Verification items for the finished model (mm, model axes). Round coordinates to 2 decimals unless told otherwise and drop trailing zeros. Order: outer loops, then holes, each group sorted by start corner. A loop starts at its lowest first (then second) coordinate and runs counter-clockwise, first axis right, second up. Notation, with made-up numbers: M 55.5,56 L 77.5,56 A19 cw 77.5,60 Z; hole C 37,-8.75 d11. An arc over 180 degrees is marked long. One line per item, written item: value. Start each with the question number.
from build123d import *

# Parameters (mm, degrees)
SKETCH009_W   = 75
SKETCH009_H   = 95
PAD005_DEPTH  = 3
SKETCH010_W   = 75
SKETCH010_H   = 95
SKETCH010_W_2 = 51.4
SKETCH010_H_2 = 20.2
SKETCH010_W_3 = 20
SKETCH010_H_3 = 92.6
SKETCH010_W_4 = 15.2
SKETCH010_H_4 = 35
SKETCH010_W_5 = 35
PAD006_DEPTH  = 30
FILLET003_R   = 1.8


with BuildPart() as part:
    # Sketch009 → Pad005 (new body)
    with BuildSketch(Plane.XZ):
        Rectangle(SKETCH009_W, SKETCH009_H)
    extrude(amount=PAD005_DEPTH)

    # Sketch010 → Pad006 (join)
    with BuildSketch(Plane.XZ.offset(2)):
        Rectangle(SKETCH010_W, SKETCH010_H)
        with Locations((-10.6, 36.2)):
            Rectangle(SKETCH010_W_2, SKETCH010_H_2, mode=Mode.SUBTRACT)
        with Locations((26.3, 0)):
            Rectangle(SKETCH010_W_3, SKETCH010_H_3, mode=Mode.SUBTRACT)
        with Locations((-28.7, 7.4)):
            Rectangle(SKETCH010_W_4, SKETCH010_H_4, mode=Mode.SUBTRACT)
        with Locations((-28.7, -28.8)):
            Rectangle(SKETCH010_W_4, SKETCH010_H_4, mode=Mode.SUBTRACT)
        with Locations((-2.4, 7.4)):
            Rectangle(SKETCH010_W_5, SKETCH010_H_4, mode=Mode.SUBTRACT)
        with Locations((-2.4, -28.8)):
            Rectangle(SKETCH010_W_5, SKETCH010_H_4, mode=Mode.SUBTRACT)
    extrude(amount=PAD006_DEPTH)

    # Fillet003
    fillet003_edges = [part.edges().sort_by_distance(p)[0] for p in [
        (0, 0, 47.5),
        (37.5, 0, 0),
        (0, 0, -47.5),
        (-37.5, 0, 0),
    ]]
    fillet(fillet003_edges, radius=FILLET003_R)


solid = part.part
1. Section check B-B (x = 30.5). Record the cut outline in (y, z), and give its area (3 significant figures).
2. Section check D-D (x = -3). Record the cut outline in (y, z), and give its area (3 significant figures).
3. Scan lines: line 1 along X through (y, z) = (-20, 8.5); line 2 along Z through (x, y) = (-29, -26); line 3 along X through (y, z) = (-12.5, 36). Record each from-to range of solid material in increasing order.
4. Section check A-A (y = -7). Record the cut outline in (x, z).
5. Depth check by flat-ended pin: pin 1 (5 mm diameter, centred on x = -3.5, z = -30.5, fed in from -Y); pin 2 (16.5 mm diameter, centred on x = -32.5, z = 8.5, fed in from -Y). Enter the tip coordinate at first touch or a pass-through.
6. Draft check along Z on faces 1 (the face through (-1, -17, -47.5)), 2 (the face through (-3, -3, 8)). Enter one of: released by +Z, released by -Z, zero draft, split by the parting line, or undercut.
7. Section check C-C (z = 13). Record the cut outline in (x, y).
Geometry check:
1. outline: M -32,-47.5 L -1.8,-47.5 A1.8 ccw 0,-45.7 L 0,45.7 A1.8 ccw -1.8,47.5 L -32,47.5 L -32,46.3 L -3,46.3 L -3,-46.3 L -32,-46.3 Z
1. area: 353 mm²
2. outline: M -32,-47.5 L -1.8,-47.5 A1.8 ccw 0,-45.7 L 0,45.7 A1.8 ccw -1.8,47.5 L -32,47.5 L -32,46.3 L -3,46.3 L -3,26.1 L -32,26.1 L -32,24.9 L -3,24.9 L -3,-10.1 L -32,-10.1 L -32,-11.3 L -3,-11.3 L -3,-46.3 L -32,-46.3 Z
2. area: 423 mm²
3. line 1: x = -37.5 to -36.3, -21.1 to -19.9, 15.1 to 16.3, 36.3 to 37.5
3. line 2: z = -47.5 to -46.3, -11.3 to -10.1, 24.9 to 26.1, 46.3 to 47.5
3. line 3: x = -37.5 to -36.3, 15.1 to 16.3, 36.3 to 37.5
4. outline: M -37.5,-47.5 L 37.5,-47.5 L 37.5,47.5 L -37.5,47.5 Z; hole M -36.3,-46.3 L -21.1,-46.3 L -21.1,-11.3 L -36.3,-11.3 Z; hole M -36.3,-10.1 L -21.1,-10.1 L -21.1,24.9 L -36.3,24.9 Z; hole M -36.3,26.1 L 15.1,26.1 L 15.1,46.3 L -36.3,46.3 Z; hole M -19.9,-46.3 L 15.1,-46.3 L 15.1,-11.3 L -19.9,-11.3 Z; hole M -19.9,-10.1 L 15.1,-10.1 L 15.1,24.9 L -19.9,24.9 Z; hole M 16.3,-46.3 L 36.3,-46.3 L 36.3,46.3 L 16.3,46.3 Z
5. pin 1: stops at y = -3
5. pin 2: stops at y = -32
6. face 1: released by -Z
6. face 2: undercut
7. outline: M -37.5,-32 L -36.3,-32 L -36.3,-3 L -21.1,-3 L -21.1,-32 L -19.9,-32 L -19.9,-3 L 15.1,-3 L 15.1,-32 L 16.3,-32 L 16.3,-3 L 36.3,-3 L 36.3,-32 L 37.5,-32 L 37.5,-1.8 A1.8 ccw 35.7,0 L -35.7,0 A1.8 ccw -37.5,-1.8 Z
